```python
from build123d import *

# Parameters (mm, degrees)
SKETCH1_R           = 2.1
SKETCH1_R_2         = 1.65
SKETCH1_R_3         = 1.7
SKETCH1_W           = 6.2
SKETCH1_H           = 10
SKETCH1_W_2         = 37
SKETCH1_H_2         = 70
BOSS_EXTRUDE1_DEPTH = 6


with BuildPart() as part:
    # Sketch1 → Boss-Extrude1 (new body)
    with BuildSketch(Plane(origin=(0, 0, 0), x_dir=(1, 0, 0), z_dir=(0, 1, 0))):
        Polygon((-90, -90), (90, -90), (90, -75), (96, -75), (96, -50), (90, -50), (90, -43.266666667), (85, -43.266666667), (85, -44.566666667), (81.8, -44.566666667), (81.8, -43.266666667), (73.8, -43.266666667), (73.8, -40.066666667), (81.8, -40.066666667), (81.8, -38.766666667), (85, -38.766666667), (85, -40.066666667), (90, -40.066666667), (90, -33.333333333), (96, -33.333333333), (96, -8.333333333), (90, -8.333333333), (90, -1.6), (85, -1.6), (85, -2.9), (81.8, -2.9), (81.8, -1.6), (73.8, -1.6), (73.8, 1.6), (81.8, 1.6), (81.8, 2.9), (85, 2.9), (85, 1.6), (90, 1.6), (90, 8.333333333), (96, 8.333333333), (96, 33.333333333), (90, 33.333333333), (90, 50), (96, 50), (96, 75), (90, 75), (90, 90), (75, 90), (75, 96), (50, 96), (50, 90), (43.266666667, 90), (43.266666667, 85), (44.566666667, 85), (44.566666667, 81.8), (43.266666667, 81.8), (43.266666667, 75), (40.066666667, 75), (40.066666667, 81.8), (38.766666667, 81.8), (38.766666667, 85), (40.066666667, 85), (40.066666667, 90), (33.333333333, 90), (33.333333333, 96), (8.333333333, 96), (8.333333333, 90), (1.6, 90), (1.6, 85), (2.9, 85), (2.9, 81.8), (1.6, 81.8), (1.6, 75), (-1.6, 75), (-1.6, 81.8), (-2.9, 81.8), (-2.9, 85), (-1.6, 85), (-1.6, 90), (-8.333333333, 90), (-8.333333333, 96), (-33.333333333, 96), (-33.333333333, 90), (-40.066666667, 90), (-40.066666667, 85), (-38.766666667, 85), (-38.766666667, 81.8), (-40.066666667, 81.8), (-40.066666667, 75), (-43.266666667, 75), (-43.266666667, 81.8), (-44.566666667, 81.8), (-44.566666667, 85), (-43.266666667, 85), (-43.266666667, 90), (-50, 90), (-50, 96), (-75, 96), (-75, 90), (-90, 90), (-90, 75), (-96, 75), (-96, 50), (-90, 50), (-90, 33.333333333), (-96, 33.333333333), (-96, 8.333333333), (-90, 8.333333333), (-90, 1.6), (-85, 1.6), (-85, 2.9), (-81.8, 2.9), (-81.8, 1.6), (-73.8, 1.6), (-73.8, -1.6), (-81.8, -1.6), (-81.8, -2.9), (-85, -2.9), (-85, -1.6), (-90, -1.6), (-90, -8.333333333), (-96, -8.333333333), (-96, -33.333333333), (-90, -33.333333333), (-90, -40.066666667), (-85, -40.066666667), (-85, -38.766666667), (-81.8, -38.766666667), (-81.8, -40.066666667), (-73.8, -40.066666667), (-73.8, -43.266666667), (-81.8, -43.266666667), (-81.8, -44.566666667), (-85, -44.566666667), (-85, -43.266666667), (-90, -43.266666667), (-90, -50), (-96, -50), (-96, -75), (-90, -75), align=None)
        with Locations(Location((65, -41, 0), (0, 0, 270))):
            Circle(SKETCH1_R, mode=Mode.SUBTRACT)
        with Locations(Location((65, -81, 0), (0, 0, 270))):
            Circle(SKETCH1_R, mode=Mode.SUBTRACT)
        with Locations(Location((-65, -81, 0), (0, 0, 90))):
            Circle(SKETCH1_R, mode=Mode.SUBTRACT)
        with Locations(Location((-65, -41, 0), (0, 0, 90))):
            Circle(SKETCH1_R, mode=Mode.SUBTRACT)
        with Locations(Location((21.75, 45.5, 0), (0, 0, 270))):
            Circle(SKETCH1_R_2, mode=Mode.SUBTRACT)
        with Locations(Location((-17.75, 45.5, 0), (0, 0, 270))):
            Circle(SKETCH1_R_2, mode=Mode.SUBTRACT)
        with Locations(Location((-17.75, 85, 0), (0, 0, 270))):
            Circle(SKETCH1_R_2, mode=Mode.SUBTRACT)
        with Locations(Location((21.75, 85, 0), (0, 0, 270))):
            Circle(SKETCH1_R_2, mode=Mode.SUBTRACT)
        with Locations(Location((-31.75, 68, 0), (0, 0, 270))):
            Circle(SKETCH1_R_2, mode=Mode.SUBTRACT)
        with Locations(Location((31.75, 68, 0), (0, 0, 270))):
            Circle(SKETCH1_R_2, mode=Mode.SUBTRACT)
        with Locations(Location((-13.770355578, 0.4, 0), (0, 0, 270))):
            Circle(SKETCH1_R_3, mode=Mode.SUBTRACT)
        with Locations(Location((13.770355578, 0.4, 0), (0, 0, 270))):
            Circle(SKETCH1_R_3, mode=Mode.SUBTRACT)
        with Locations(Location((64.229644422, 0.4, 0), (0, 0, 270))):
            Circle(SKETCH1_R_3, mode=Mode.SUBTRACT)
        with Locations(Location((-64.229644422, 0.4, 0), (0, 0, 270))):
            Circle(SKETCH1_R_3, mode=Mode.SUBTRACT)
        with Locations((26.9, 19.4)):
            Rectangle(SKETCH1_W, SKETCH1_H, mode=Mode.SUBTRACT)
        with Locations((65.5, 40)):
            Rectangle(SKETCH1_W_2, SKETCH1_H_2, mode=Mode.SUBTRACT)
        with Locations((-65.5, 40)):
            Rectangle(SKETCH1_W_2, SKETCH1_H_2, mode=Mode.SUBTRACT)
        with Locations((-26.9, 19.4)):
            Rectangle(SKETCH1_W, SKETCH1_H, mode=Mode.SUBTRACT)
        with BuildLine():
            Line((-40.5, -35), (-40.5, -55))
            ThreePointArc((-40.5, -55), (-42, -56.5), (-43.5, -55))
            Line((-43.5, -55), (-43.5, -35))
            ThreePointArc((-43.5, -35), (-42, -33.5), (-40.5, -35))
        make_face(mode=Mode.SUBTRACT)
        with BuildLine():
            Line((40.5, -35), (40.5, -55))
            ThreePointArc((40.5, -55), (42, -56.5), (43.5, -55))
            Line((43.5, -55), (43.5, -35))
            ThreePointArc((43.5, -35), (42, -33.5), (40.5, -35))
        make_face(mode=Mode.SUBTRACT)
        with BuildLine():
            Line((10, -12), (-10, -12))
            ThreePointArc((-10, -12), (-11.5, -10.5), (-10, -9))
            Line((-10, -9), (10, -9))
            ThreePointArc((10, -9), (11.5, -10.5), (10, -12))
        make_face(mode=Mode.SUBTRACT)
        with BuildLine():
            Line((10, -78), (-10, -78))
            ThreePointArc((-10, -78), (-11.5, -79.5), (-10, -81))
            Line((-10, -81), (10, -81))
            ThreePointArc((10, -81), (11.5, -79.5), (10, -78))
        make_face(mode=Mode.SUBTRACT)
    extrude(amount=BOSS_EXTRUDE1_DEPTH)


solid = part.part
```
The model under review builds one solid part; all positions refer to its coordinate system, in mm. A direction names the side the tool comes from. Round coordinates to 2 decimals unless told otherwise and drop trailing zeros. Order: outer loops, then holes, each group sorted by start corner. A loop starts at its lowest first (then second) coordinate and runs counter-clockwise, first axis right, second up. Notation, with made-up numbers: (70.5, 9.5) -> (118.5, 9.5) arc R17 ccw to (118.5, 25.5) -> close; hole circle Ø5 at (56, 70.5). An arc over 180 degrees is marked (long way). One line per item, written item: value. Start each with the question number.
Q1. Machinability: for faces 5 (the face through (50, 3, -93)), 6 (the face through (-30, 3, -19)), 7 (the face through (93, 3, 8.333)), 8 (the face through (-90, 3, 47)), which of the approach directions +Z, -Z, +X, -X, +Y, -Y give a long, thin tool a straight path to every point of the face, cutting with its end or side? Answer none if there is none.
Q2. Take a section at D-D (z = -54). Write out the cut boundary in (x, y).
Q3. Take a section at A-A (x = 78). Write out the cut boundary in (y, z).
Q4. Take a section at B-B (z = -21). Write out the cut boundary in (x, y).
Q5. Wall thickness on line 1 (X direction, y = 4.85, z = -7); line 2 (X direction, y = 4.7, z = 38); line 3 (X direction, y = 3.8, z = -45.5): over which ranges is each line inside the solid? List them lowest first.
Q6. Take a section at C-C (x = -26). Write out the cut boundary in (y, z).
Q7. Clearance check with flat-ended pins moving along their axes: pin 1 Ø1.8 at (x, y) = (-91.5, 4) entering from -Z; pin 2 Ø4 at (x, z) = (-17.75, -45.5) entering from -Y; pin 3 Ø0.6 at (y, z) = (2, 39.5) entering from +X; pin 4 Ø1.8 at (y, z) = (2, -91.5) entering from +X. State where each tip first meets the part, or that it passes through.
Q8. Mouldability with a two-part tool opening along X and no side actions: class faces 1 (the face through (-90, 3, 5)), 2 (the face through (-5, 3, -90)), 3 (the face through (90, 3, 5)), 4 (the face through (88, 3, 43.267)) as released by +X, released by -X, zero draft, split by the parting line, or undercut.
Reported:
1. face 5: -Z, +Y, -Y
1. face 6: +Y, -Y
1. face 7: +X, +Y, -Y
1. face 8: -X, +Y, -Y
2. outline: (-96, 0) -> (-84, 0) -> (-84, 6) -> (-96, 6) -> close; (-47, 0) -> (47, 0) -> (47, 6) -> (-47, 6) -> close; (84, 0) -> (96, 0) -> (96, 6) -> (84, 6) -> close
3. outline: (0, -90) -> (6, -90) -> (6, -75) -> (0, -75) -> close; (0, -5) -> (6, -5) -> (6, -1.6) -> (0, -1.6) -> close; (0, 1.6) -> (6, 1.6) -> (6, 40.07) -> (0, 40.07) -> close; (0, 43.27) -> (6, 43.27) -> (6, 90) -> (0, 90) -> close
4. outline: (-96, 0) -> (-84, 0) -> (-84, 6) -> (-96, 6) -> close; (-47, 0) -> (-30, 0) -> (-30, 6) -> (-47, 6) -> close; (-23.8, 0) -> (23.8, 0) -> (23.8, 6) -> (-23.8, 6) -> close; (30, 0) -> (47, 0) -> (47, 6) -> (30, 6) -> close; (84, 0) -> (96, 0) -> (96, 6) -> (84, 6) -> close
5. line 1: x = -90 to -84, -47 to 47, 84 to 90
5. line 2: x = -90 to -43.5, -40.5 to 40.5, 43.5 to 90
5. line 3: x = -90 to -84, -47 to -19.4, -16.1 to 20.1, 23.4 to 47, 84 to 90
6. outline: (0, -96) -> (6, -96) -> (6, -24.4) -> (0, -24.4) -> close; (0, -14.4) -> (6, -14.4) -> (6, 90) -> (0, 90) -> close
7. pin 1: stops at z = -75
7. pin 2: stops at y = 0
7. pin 3: stops at x = 90
7. pin 4: stops at x = 75
8. face 1: released by -X
8. face 2: undercut
8. face 3: released by +X
8. face 4: zero draft
